Read the model definition and answer for the solid it produces. Units are mm, in the model's axes. A direction names the side the tool comes from. Round coordinates to 2 decimals unless told otherwise and drop trailing zeros. Order: outer loops, then holes, each group sorted by start corner. A loop starts at its lowest first (then second) coordinate and runs counter-clockwise, first axis right, second up. Notation, with made-up numbers: (-39, 35.5) -> (16, 35.5) arc R11 ccw to (16, 48.5) -> close; hole circle Ø6 at (56.25, -25). An arc over 180 degrees is marked (long way). Answer as a JSON object with one key per item and string values. Group by question number.
Item 1: Section A-A, the plane x = 6 is taken. Write down the section's boundary in (y, z).
Item 2: Section C-C, the plane y = 0 is taken. Write down the section's boundary in (x, z), plus the area to 3 significant figures.
Item 3: The mould has two halves that part along Z. Classify faces 1 (the flat face through (5, 0, 17)), 2 (the cylindrical face through (-0.29, 2.23, 30.01)), 3 (the flat face through (0, 7, 28)): pulls with the +Z half, pulls with the -Z half, needs draft (parallel to the pull), parting line crosses it, or undercut.
Item 4: Section D-D, the plane z = 13.25 is taken. Write down the section's boundary in (x, y).
Item 5: For faces 4 (the flat face through (-1, 6, 19)), 5 (the flat face through (6, -1, 21)), 6 (the flat face through (-6, -1, 19)), 7 (the flat face through (6, 0, 14)), determine the directions among +Z, -Z, +X, -X, +Y, -Y from which every point of the face is accessible in a straight line to the end or side of a thin tool.
Item 6: Given P1, Ø5.5, axis at x = 6, z = 23, coming from the +Y side; P2, Ø4, axis at y = 7.5, z = 16.5, coming from the +X side; P3, Ø5.5, axis at x = 5.5, z = 17, coming from the -Y side; P4, Ø4, axis at x = 0, y = 0, coming from the +Z side, each flat-ended and moving along its own axis, determine where each tip first touches the part or whether it passes through.
Item 7: Consider probe 1 along Y at (x, z) = (0, 16.25); probe 2 along Y at (x, z) = (-8, 14.25); probe 3 along Z at (x, y) = (-1.5, -2.75). Determine where each line is inside the solid, lowest interval first. Write a range as from..to.
Item 8: Section B-B, the plane z = 15.75 is taken. Write down the section's boundary in (x, y), plus the area to 3 significant figures.
from build123d import *

# Parameters (mm, degrees)
PAD_DEPTH            = 20
SKETCH001_W          = 2.5
SKETCH001_H          = 6
POCKET_DEPTH         = 10.001
SKETCH002_R          = 3.25
POCKET001_DEPTH      = 18
SKETCH003_R          = 2.25
POCKET002_DEPTH      = 2
CHAMFER_SIZE         = 5
BODY_PLACEMENT_ANGLE = 180


with BuildPart() as part:
    # Sketch → Pad (new body)
    with BuildSketch(Plane.XY):
        with BuildLine():
            ThreePointArc((-3.872983, -1), (-2.828427, -2.828427), (-1, -3.872983))
            Line((-1, -9), (-1, -3.872983))
            Line((1, -9), (-1, -9))
            Line((1, -3.872983), (1, -9))
            ThreePointArc((1, -3.872983), (2.828427, -2.828427), (3.872983, -1))
            Line((9, -1), (3.872983, -1))
            Line((9, 1), (9, -1))
            Line((3.872983, 1), (9, 1))
            ThreePointArc((3.872983, 1), (2.828427, 2.828427), (1, 3.872983))
            Line((1, 9), (1, 3.872983))
            Line((-1, 9), (1, 9))
            Line((-1, 3.872983), (-1, 9))
            ThreePointArc((-1, 3.872983), (-2.828427, 2.828427), (-3.872983, 1))
            Line((-9, 1), (-3.872983, 1))
            Line((-9, -1), (-9, 1))
            Line((-3.872983, -1), (-9, -1))
        make_face()
    extrude(amount=PAD_DEPTH)

    # Sketch001 (on Face6 of Pad) → Pocket (cut, through all)
    with BuildSketch(Plane.XZ.offset(1)):
        with Locations((6.25, 14)):
            Rectangle(SKETCH001_W, SKETCH001_H)
    extrude(amount=-POCKET_DEPTH, mode=Mode.SUBTRACT)

    # Sketch002 (on Face5 of Pocket) → Pocket001 (cut)
    with BuildSketch(Plane.XY.offset(20)):
        Circle(SKETCH002_R)
    extrude(amount=-POCKET001_DEPTH, mode=Mode.SUBTRACT)

    # Sketch003 (on Face4 of Pocket001) → Pocket002 (cut)
    with BuildSketch(Plane(origin=(0, 0, 0), x_dir=(1, 0, 0), z_dir=(0, 0, -1))):
        Circle(SKETCH003_R)
    extrude(amount=-POCKET002_DEPTH, mode=Mode.SUBTRACT)

    # Chamfer
    chamfer_edges = [part.edges().sort_by_distance(p)[0] for p in [
        (-9, 0, 0),
        (0, -9, 0),
        (9, 0, 0),
        (0, 9, 0),
    ]]
    chamfer(chamfer_edges, length=CHAMFER_SIZE)


with BuildPart() as part_1:
    # Body placement: moved
    add(part.part.moved(Location((0, 0, 31))).rotate(Axis((0, 0, 31), (1, 0, 0)), BODY_PLACEMENT_ANGLE))


solid = part_1.part
Values found:
{
 "1": {"outline": "(-1, 11) -> (1, 11) -> (1, 14) -> (-1, 14) -> close; (-1, 20) -> (1, 20) -> (1, 29) -> (-1, 29) -> close"},
 "2": {"outline": "(-9, 11) -> (-3.25, 11) -> (-3.25, 29) -> (-2.25, 29) -> (-2.25, 31) -> (-4, 31) -> (-9, 26) -> close; (2.25, 29) -> (3.25, 29) -> (3.25, 11) -> (9, 11) -> (9, 26) -> (4, 31) -> (2.25, 31) -> close; hole (5, 14) -> (7.5, 14) -> (7.5, 20) -> (5, 20) -> close", "area": "194 mm2"},
 "3": {"face 1": "undercut", "face 2": "needs draft", "face 3": "pulls with the +Z half"},
 "4": {"outline": "(-9, -1) -> (-3.87, -1) arc R4 ccw to (-1, -3.87) -> (-1, -9) -> (1, -9) -> (1, -3.87) arc R4 ccw to (3.87, -1) -> (9, -1) -> (9, 1) -> (3.87, 1) arc R4 ccw to (1, 3.87) -> (1, 9) -> (-1, 9) -> (-1, 3.87) arc R4 ccw to (-3.87, 1) -> (-9, 1) -> close; hole circle Ø6.5 at (0, 0)"},
 "5": {"face 4": "+Z, -Z, -X, +Y", "face 5": "+Z, -Z, +X, -Y", "face 6": "+Z, -Z, -X, -Y", "face 7": "+Y, -Y"},
 "6": {"P1": "y = 2.33", "P2": "x = 1", "P3": "y = -2.9", "P4": "through"},
 "7": {"probe 1": "-9..-3.25, 3.25..9", "probe 2": "-1..1", "probe 3": "29..31"},
 "8": {"outline": "(-9, -1) -> (-3.87, -1) arc R4 ccw to (-1, -3.87) -> (-1, -9) -> (1, -9) -> (1, -3.87) arc R4 ccw to (3.87, -1) -> (5, -1) -> (5, 1) -> (3.87, 1) arc R4 ccw to (1, 3.87) -> (1, 9) -> (-1, 9) -> (-1, 3.87) arc R4 ccw to (-3.87, 1) -> (-9, 1) -> close; (7.5, -1) -> (9, -1) -> (9, 1) -> (7.5, 1) -> close; hole circle Ø6.5 at (0, 0)", "area": "52.4 mm2"}
}
